Input: part model. Units: mm. Frame: model coordinates. A direction names the side the tool comes from. Coordinates: 2 decimals unless noted, no trailing zeros. Write each loop counter-clockwise with the first axis right and the second up, starting at its lowest first coordinate (ties: lowest second). Pieces come first, ordered by that corner, then holes. Notation, with made-up numbers: M -40,-16.5 L 18,-16.5 A7 ccw 18,-4.5 Z; hole C 30,80 d5. An arc over 180 degrees is marked long. Write each question's results on one line, items separated by ' | '. Start each with the question number.
1. Set-up query: faces 1 (the flat face through (1.6, -1.3, -0.2)), 2 (the flat face through (1.4, -1.3, 0.2)), 3 (the flat face through (0, 4, 1.27)). Return all of +Z, -Z, +X, -X, +Y, -Y with unobstructed straight access to the full face (end or side cutting, diameter ignored); none if empty.
2. First-contact query: pin 1 (3 mm diameter, centred on x = 4, y = 0, fed in from +Z). Flat tip, straight axial feed; report the tip coordinate or a pass-through.
3. Section query B-B, the plane z = 0.45. Output: boundary loops of the cut face in (x, y), and give its area (3 significant figures).
4. Section query C-C, the plane x = -0.35. Output: boundary loops of the cut face in (y, z).
5. Ray query, probe 1 along X at (y, z) = (6.25, -0.6); probe 2 along Y at (x, z) = (1.15, -0.45); probe 3 along Y at (x, z) = (0.3, -0.55). Return the intervals inside material, ascending.
6. Section query D-D, the plane y = 2. Output: boundary loops of the cut face in (x, z).
7. Section query A-A, the plane y = 5. Output: boundary loops of the cut face in (x, z).
Autodesk Inventor part; units mm, degrees
ref_plane "YZ Plane" through (0, 0, 0) normal (1, 0, 0) x (0, 1, 0)
ref_plane "XZ Plane" through (0, 0, 0) normal (0, 1, 0) x (-1, 0, 0)
ref_plane "XY Plane" through (0, 0, 0) normal (0, 0, 1) x (1, 0, 0)
sketch "Sketch1" plane through (0, 0, 0) normal (0, 1, 0) x (-1, 0, 0)
  line L0 (-1.27, 1.27) -> (1.27, 1.27)
  line L1 (1.27, 1.27) -> (1.27, -1.27)
  line L2 (1.27, -1.27) -> (-1.27, -1.27)
  line L3 (-1.27, -1.27) -> (-1.27, 1.27)
  line L4 (-1.27, 1.27) -> (1.27, -1.27) construction
  line L5 (1.27, 1.27) -> (-1.27, -1.27) construction
  point P0 (0, 0)
  dimension "d0" = 2.54
  dimension "d1" = 2.54
extrude "Extrusion1" add sketch "Sketch1" along normal blind 8.5
sketch "Sketch2" plane through (0, 8.5, 0) normal (0, 1, 0) x (1, 0, 0)
  line L0 (0.2, -0.2) -> (-0.2, -0.2)
  line L1 (-0.2, -0.2) -> (-0.2, 0.2)
  line L2 (-0.2, 0.2) -> (0.2, 0.2)
  line L3 (0.2, 0.2) -> (0.2, -0.2)
  line L4 (0.2, -0.2) -> (-0.2, 0.2) construction
  line L5 (-0.2, -0.2) -> (0.2, 0.2) construction
  point P0 (0, 0)
  dimension "d4" = 0.4
  dimension "d5" = 0.4
extrude "Extrusion2" cut sketch "Sketch2" against normal blind 5
chamfer "Chamfer1" distance 0.75 angle 45 4 edges at (0, 8.5, 0.2) (-0.2, 8.5, 0) (0, 8.5, -0.2) (0.2, 8.5, 0)
sketch "Sketch3" plane through (0, 0, 0) normal (0, -1, 0) x (1, 0, 0)
  line L0 (-0.2, 0.2) -> (0.2, 0.2)
  line L1 (0.2, 0.2) -> (0.2, -0.2)
  line L2 (0.2, -0.2) -> (-0.2, -0.2)
  line L3 (-0.2, -0.2) -> (-0.2, 0.2)
  line L4 (-0.2, 0.2) -> (0.2, -0.2) construction
  line L5 (0.2, 0.2) -> (-0.2, -0.2) construction
  point P0 (0, 0)
  dimension "d11" = 0.4
  dimension "d12" = 0.4
extrude "Extrusion3" add sketch "Sketch3" along normal blind 1.5
sketch "Sketch4" plane through (-0.2, 0, 0.2) normal (0, 0, 1) x (1, 0, 0)
  line L0 (0, -1.5) -> (4.75, -1.5)
  line L1 (4.75, -1.5) -> (4.75, -1.1)
  line L2 (4.75, -1.1) -> (0, -1.1)
  line L3 (0, -1.1) -> (0, -1.5)
  point P0 (0.2, 0)
  dimension "d27" = 0.4
  dimension "d28" = 4.75
extrude "Extrusion4" add sketch "Sketch4" against normal up to surface (0.4 mm away)
fillet "Fillet1" radius 0.5 1 edges at (-0.2, -1.5, 0)
fillet "Fillet2" radius 0.15 1 edges at (0.2, -1.1, 0)
chamfer "Chamfer6" distance 0.5 distance2 0.1 1 edges at (4.55, -1.3, 0.2) measured on face at (1.7333, -1.3667, 0.2)
chamfer "Chamfer7" distance 0.5 distance2 0.1 1 edges at (4.55, -1.1, -0.05) measured on face at (2.9833, -1.1, -0.0667)
chamfer "Chamfer8" distance 0.1 distance2 0.5 1 edges at (4.55, -1.35, -0.2) measured on face at (4.55, -1.4, 0)
chamfer "Chamfer9" distance 0.1 distance2 0.5 1 edges at (4.55, -1.5, 0) measured on face at (4.55, -1.4, 0.0333)
properties part number "FemaleHederPin_90"
Answer:
1) face 1: -Z, +X, -X, -Y | face 2: +Z, +X, -X, -Y | face 3: +Z, +X, -X, +Y, -Y
2) pin 1: z = 0.2
3) outline: M -1.27,0 L 1.27,0 L 1.27,8.5 L 0.95,8.5 L 0.45,8 L -0.45,8 L -0.95,8.5 L -1.27,8.5 Z | area: 20.9 mm^2
4) outline: M 0,-1.27 L 8.5,-1.27 L 8.5,-0.95 L 7.9,-0.35 L 7.9,0.35 L 8.5,0.95 L 8.5,1.27 L 0,1.27 Z
5) probe 1: -1.27 to 1.27 | probe 2: 0 to 8.5 | probe 3: 0 to 8.1
6) outline: M -1.27,-1.27 L 1.27,-1.27 L 1.27,1.27 L -1.27,1.27 Z
7) outline: M -1.27,-1.27 L 1.27,-1.27 L 1.27,1.27 L -1.27,1.27 Z; hole M -0.2,-0.2 L 0.2,-0.2 L 0.2,0.2 L -0.2,0.2 Z
